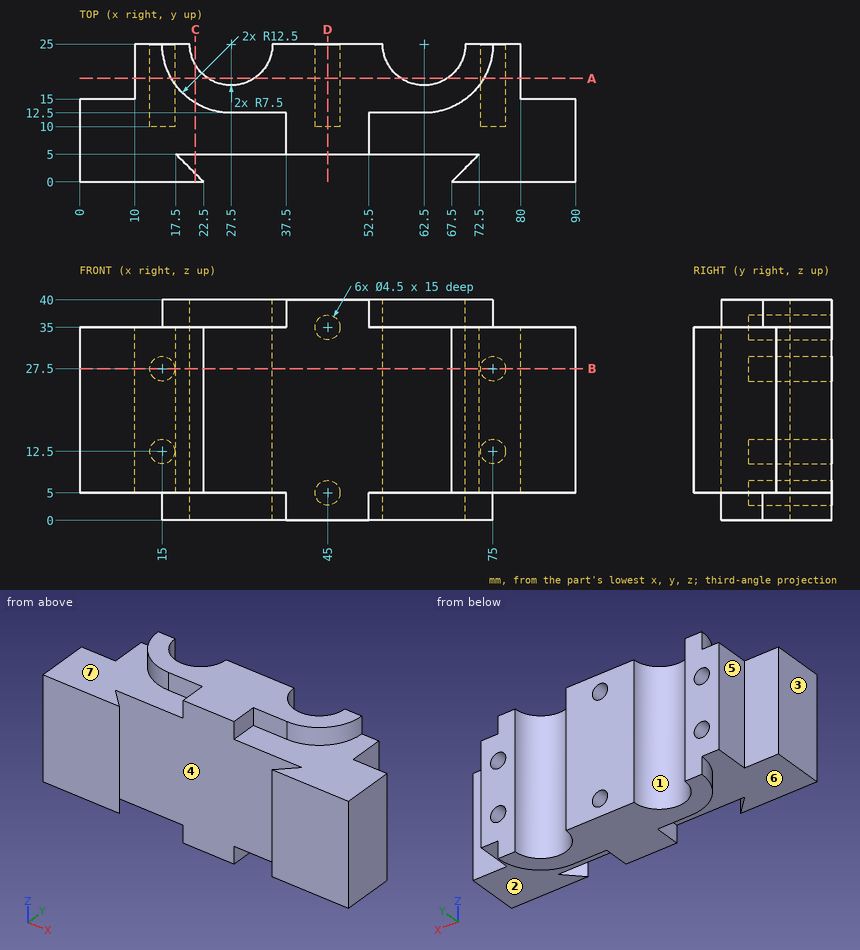
Geometry check sheet. Reference: drawing and pictorial views, mm from the part's lowest x, y, z. A direction names the side the tool comes from. Round coordinates to 2 decimals unless told otherwise and drop trailing zeros. Write each loop counter-clockwise with the first axis right and the second up, starting at its lowest first coordinate (ties: lowest second). Pieces come first, ordered by that corner, then holes. Notation, with made-up numbers: (74, 23) -> (123, 23) arc R29 ccw to (123, 61) -> close; hole circle Ø4 at (52.5, -30). An arc over 180 degrees is marked (long way). Put each result on its own line as item: value.
1) Cross-section at D-D, the plane x = 45. Enter the section's corners in (y, z), plus the area to 3 significant figures.
Recorded:
outline: (5, 0) -> (25, 0) -> (25, 2.75) -> (10, 2.75) -> (10, 7.25) -> (25, 7.25) -> (25, 32.75) -> (10, 32.75) -> (10, 37.25) -> (25, 37.25) -> (25, 40) -> (5, 40) -> close
area: 665 mm2
2) Cross-section at C-C, the plane x = 21. Enter the section's corners in (y, z).
Recorded:
outline: (0, 5) -> (1.5, 5) -> (1.5, 35) -> (0, 35) -> close; (5, 5) -> (14.32, 5) -> (14.32, 0) -> (21.26, 0) -> (21.26, 40) -> (14.32, 40) -> (14.32, 35) -> (5, 35) -> close
3) Release check for a two-part mould opening along X. For the marked faces 1, 2 and 3 record: pulls with the +X half, pulls with the -X half, needs draft (parallel to the pull), parting line crosses it, or undercut.
Recorded:
face 1: undercut
face 2: needs draft
face 3: pulls with the -X half
4) Cross-section at B-B, the plane z = 27.5. Enter the section's corners in (x, y), plus the area to 3 significant figures.
Recorded:
outline: (0, 0) -> (22.5, 0) -> (17.5, 5) -> (72.5, 5) -> (67.5, 0) -> (90, 0) -> (90, 15) -> (80, 15) -> (80, 25) -> (77.25, 25) -> (77.25, 10) -> (72.75, 10) -> (72.75, 25) -> (70, 25) arc R7.5 cw to (55, 25) -> (35, 25) arc R7.5 cw to (20, 25) -> (17.25, 25) -> (17.25, 10) -> (12.75, 10) -> (12.75, 25) -> (10, 25) -> (10, 15) -> (0, 15) -> close
area: 1,490 mm2
5) Access from +Z, -Z, +X, -X, +Y, -Y to the whole of each face (thin tool, end or side, straight path). Record for the marked faces 4, 5, 6 and 7.
Recorded:
face 4: +Z, -Z
face 5: +Z, -Z, -X, +Y
face 6: -Z, -X, -Y
face 7: +Z, -X, -Y
6) Thickness scan on probe 1 along Z at (x, y) = (45, 21.75); probe 2 along Z at (x, y) = (75, 13.5); probe 3 along X at (y, z) = (17, 12.5). Record the ranges inside material, lowest first. Write a range as from..to.
Recorded:
probe 1: z = 0..2.75, 7.25..32.75, 37.25..40
probe 2: z = 5..10.25, 14.75..25.25, 29.75..35
probe 3: x = 10..12.75, 17.25..72.75, 77.25..80
7) Cross-section at A-A, the plane y = 18.75. Give the number of separate pieces and of enclosed holes in the cut face, plus the area to 3 significant figures.
Recorded:
separate pieces: 3
enclosed holes: 6
area: 1,910 mm2
8) Depth check by flat-ended pin: P1, Ø5, axis at y = 21.5, z = 14, coming from the -X side; P2, Ø2, axis at x = 45, z = 4, coming from the +Y side; P3, Ø4, axis at x = 35, z = 1.5, coming from the -Y side; P4, Ø5, axis at x = 49, y = 3.5, coming from the -Z side. Enter the tip coordinate at first touch or a pass-through.
Recorded:
P1: stops at x = 10
P2: stops at y = 10
P3: stops at y = 12.5
P4: stops at z = 0
